Part model, mm, in its own coordinate system. Coordinates: 2 decimals unless noted, no trailing zeros. Write item = value, one per line.
from build123d import *

# Parameters (mm, degrees)
BOSS_EXTRUDE1_DEPTH = 452


with BuildPart() as part:
    # Sketch1 → Boss-Extrude1 (new, symmetric)
    with BuildSketch(Plane.XY):
        with BuildLine():
            Line((0, -5.55), (0.25, -5.8))
            Line((0.25, -5.8), (4.385786438, -5.8))
            Line((4.385786438, -5.8), (8.2, -9.614213562))
            Line((8.2, -9.614213562), (8.2, -12.8))
            Line((8.2, -12.8), (4.1, -12.8))
            Line((4.1, -12.8), (4.1, -13.9))
            Line((4.1, -13.9), (5.2, -13.9))
            Line((5.2, -13.9), (5.2, -15))
            Line((5.2, -15), (13, -15))
            ThreePointArc((13, -15), (14.414213562, -14.414213562), (15, -13))
            Line((15, -13), (15, -5.2))
            Line((15, -5.2), (13.9, -5.2))
            Line((13.9, -5.2), (13.9, -4.1))
            Line((13.9, -4.1), (12.8, -4.1))
            Line((12.8, -4.1), (12.8, -8.2))
            Line((12.8, -8.2), (9.614213562, -8.2))
            Line((9.614213562, -8.2), (5.8, -4.385786438))
            Line((5.8, -4.385786438), (5.8, -0.25))
            Line((5.8, -0.25), (5.55, 0))
            Line((5.55, 0), (5.8, 0.25))
            Line((5.8, 0.25), (5.8, 4.385786438))
            Line((5.8, 4.385786438), (9.614213562, 8.2))
            Line((9.614213562, 8.2), (12.8, 8.2))
            Line((12.8, 8.2), (12.8, 4.1))
            Line((12.8, 4.1), (13.9, 4.1))
            Line((13.9, 4.1), (13.9, 5.2))
            Line((13.9, 5.2), (15, 5.2))
            Line((15, 5.2), (15, 13))
            ThreePointArc((15, 13), (14.414213562, 14.414213562), (13, 15))
            Line((13, 15), (5.2, 15))
            Line((5.2, 15), (5.2, 13.9))
            Line((5.2, 13.9), (4.1, 13.9))
            Line((4.1, 13.9), (4.1, 12.8))
            Line((4.1, 12.8), (8.2, 12.8))
            Line((8.2, 12.8), (8.2, 9.614213562))
            Line((8.2, 9.614213562), (4.385786438, 5.8))
            Line((4.385786438, 5.8), (0.25, 5.8))
            Line((0.25, 5.8), (0, 5.55))
            Line((0, 5.55), (-0.25, 5.8))
            Line((-0.25, 5.8), (-4.385786438, 5.8))
            Line((-4.385786438, 5.8), (-8.2, 9.614213562))
            Line((-8.2, 9.614213562), (-8.2, 12.8))
            Line((-8.2, 12.8), (-4.1, 12.8))
            Line((-4.1, 12.8), (-4.1, 13.9))
            Line((-4.1, 13.9), (-5.2, 13.9))
            Line((-5.2, 13.9), (-5.2, 15))
            Line((-5.2, 15), (-13, 15))
            ThreePointArc((-13, 15), (-14.414213562, 14.414213562), (-15, 13))
            Line((-15, 13), (-15, 5.2))
            Line((-15, 5.2), (-13.9, 5.2))
            Line((-13.9, 5.2), (-13.9, 4.1))
            Line((-13.9, 4.1), (-12.8, 4.1))
            Line((-12.8, 4.1), (-12.8, 8.2))
            Line((-12.8, 8.2), (-9.614213562, 8.2))
            Line((-9.614213562, 8.2), (-5.8, 4.385786438))
            Line((-5.8, 4.385786438), (-5.8, 0.25))
            Line((-5.8, 0.25), (-5.55, 0))
            Line((-5.55, 0), (-5.8, -0.25))
            Line((-5.8, -0.25), (-5.8, -4.385786438))
            Line((-5.8, -4.385786438), (-9.614213562, -8.2))
            Line((-9.614213562, -8.2), (-12.8, -8.2))
            Line((-12.8, -8.2), (-12.8, -4.1))
            Line((-12.8, -4.1), (-13.9, -4.1))
            Line((-13.9, -4.1), (-13.9, -5.2))
            Line((-13.9, -5.2), (-15, -5.2))
            Line((-15, -5.2), (-15, -13))
            ThreePointArc((-15, -13), (-14.414213562, -14.414213562), (-13, -15))
            Line((-13, -15), (-5.2, -15))
            Line((-5.2, -15), (-5.2, -13.9))
            Line((-5.2, -13.9), (-4.1, -13.9))
            Line((-4.1, -13.9), (-4.1, -12.8))
            Line((-4.1, -12.8), (-8.2, -12.8))
            Line((-8.2, -12.8), (-8.2, -9.614213562))
            Line((-8.2, -9.614213562), (-4.385786438, -5.8))
            Line((-4.385786438, -5.8), (-0.25, -5.8))
            Line((-0.25, -5.8), (0, -5.55))
        make_face()
        with BuildLine():
            Line((-13.5, 10.7), (-13.5, 12.5))
            ThreePointArc((-13.5, 12.5), (-13.207106781, 13.207106781), (-12.5, 13.5))
            Line((-12.5, 13.5), (-10.7, 13.5))
            ThreePointArc((-10.7, 13.5), (-9.992893219, 13.207106781), (-9.7, 12.5))
            Line((-9.7, 12.5), (-9.7, 10.7))
            ThreePointArc((-9.7, 10.7), (-9.992893219, 9.992893219), (-10.7, 9.7))
            Line((-10.7, 9.7), (-12.5, 9.7))
            ThreePointArc((-12.5, 9.7), (-13.207106781, 9.992893219), (-13.5, 10.7))
        make_face(mode=Mode.SUBTRACT)
        with BuildLine():
            Line((-13.5, -12.5), (-13.5, -10.7))
            ThreePointArc((-13.5, -10.7), (-13.207106781, -9.992893219), (-12.5, -9.7))
            Line((-12.5, -9.7), (-10.7, -9.7))
            ThreePointArc((-10.7, -9.7), (-9.992893219, -9.992893219), (-9.7, -10.7))
            Line((-9.7, -10.7), (-9.7, -12.5))
            ThreePointArc((-9.7, -12.5), (-9.992893219, -13.207106781), (-10.7, -13.5))
            Line((-10.7, -13.5), (-12.5, -13.5))
            ThreePointArc((-12.5, -13.5), (-13.207106781, -13.207106781), (-13.5, -12.5))
        make_face(mode=Mode.SUBTRACT)
        with BuildLine():
            Line((13.5, -10.7), (13.5, -12.5))
            ThreePointArc((13.5, -12.5), (13.207106781, -13.207106781), (12.5, -13.5))
            Line((12.5, -13.5), (10.7, -13.5))
            ThreePointArc((10.7, -13.5), (9.992893219, -13.207106781), (9.7, -12.5))
            Line((9.7, -12.5), (9.7, -10.7))
            ThreePointArc((9.7, -10.7), (9.992893219, -9.992893219), (10.7, -9.7))
            Line((10.7, -9.7), (12.5, -9.7))
            ThreePointArc((12.5, -9.7), (13.207106781, -9.992893219), (13.5, -10.7))
        make_face(mode=Mode.SUBTRACT)
        with BuildLine():
            Line((13.5, 12.5), (13.5, 10.7))
            ThreePointArc((13.5, 10.7), (13.207106781, 9.992893219), (12.5, 9.7))
            Line((12.5, 9.7), (10.7, 9.7))
            ThreePointArc((10.7, 9.7), (9.992893219, 9.992893219), (9.7, 10.7))
            Line((9.7, 10.7), (9.7, 12.5))
            ThreePointArc((9.7, 12.5), (9.992893219, 13.207106781), (10.7, 13.5))
            Line((10.7, 13.5), (12.5, 13.5))
            ThreePointArc((12.5, 13.5), (13.207106781, 13.207106781), (13.5, 12.5))
        make_face(mode=Mode.SUBTRACT)
        with BuildLine():
            Line((-1.590718277, -3.00493184), (-3.181708535, -4.595922097))
            Line((-3.181708535, -4.595922097), (-4.595922097, -3.181708535))
            Line((-4.595922097, -3.181708535), (-3.00493184, -1.590718277))
            ThreePointArc((-3.00493184, -1.590718277), (-3.4, 0), (-3.00493184, 1.590718277))
            Line((-3.00493184, 1.590718277), (-4.595922097, 3.181708535))
            Line((-4.595922097, 3.181708535), (-3.181708535, 4.595922097))
            Line((-3.181708535, 4.595922097), (-1.590718277, 3.00493184))
            ThreePointArc((-1.590718277, 3.00493184), (0, 3.4), (1.590718277, 3.00493184))
            Line((1.590718277, 3.00493184), (3.181708535, 4.595922097))
            Line((3.181708535, 4.595922097), (4.595922097, 3.181708535))
            Line((4.595922097, 3.181708535), (3.00493184, 1.590718277))
            ThreePointArc((3.00493184, 1.590718277), (3.4, 0), (3.00493184, -1.590718277))
            Line((3.00493184, -1.590718277), (4.595922097, -3.181708535))
            Line((4.595922097, -3.181708535), (3.181708535, -4.595922097))
            Line((3.181708535, -4.595922097), (1.590718277, -3.00493184))
            ThreePointArc((1.590718277, -3.00493184), (0, -3.4), (-1.590718277, -3.00493184))
        make_face(mode=Mode.SUBTRACT)
    extrude(amount=BOSS_EXTRUDE1_DEPTH, both=True)


solid = part.part
Q1. Probe line 1 (X direction, y = 10.75, z = -92); line 2 (Y direction, x = -10.25, z = 92). List the from-to ranges inside material, lowest first. Write a range as from..to.
Model answer:
line_1 = -15..-13.5, -9.7..-8.2, 8.2..9.7, 13.5..15
line_2 = -15..-13.39, -9.81..-8.2, 8.2..9.81, 13.39..15
Q2. Pin check, flat tips, straight feed: pin 1 (0.9 mm diameter, centred on x = -14.5, z = -180, fed in from -Y); pin 2 (0.6 mm diameter, centred on y = 5, z = -59, fed in from -X); pin 3 (1.2 mm diameter, centred on y = -2, z = 84.5, fed in from -X); pin 4 (8 mm diameter, centred on y = -1, z = -109, fed in from -X). Stop position of each tip, or through.
Model answer:
pin_1 = -14.7
pin_2 = -15
pin_3 = -5.8
pin_4 = -13.9
Q3. Saw through at A-A on z = -174.5. Count the separate pieces of the cut face and the enclosed holes in it, and give its area (3 significant figures).
Model answer:
separate_pieces = 1
enclosed_holes = 5
area = 306 mm²
